Verification items for the finished model (mm, model axes). A direction names the side the tool comes from. Coordinates: 2 decimals unless noted, no trailing zeros. Loops run counter-clockwise (first coordinate to the right, second up) from the corner with the lowest first, then second, coordinate; pieces in that order, holes last.
Q1. Sectioned sample at D-D (y = 38). Enter the section's corners in (x, z).
Q2. Sectioned sample at B-B (x = 57). Enter the section's corners in (y, z).
Q3. Mould release check, pull along Y, two halves, no side actions. Record for faces 1 (the face through (58.49, 57.63, 1.48)), 2 (the face through (1, 2, 0)): +Y half, -Y half, draft (parallel to the pull), parting line (faces both ways), or undercut.
Q4. Sectioned sample at A-A (z = 0.5). Enter the section's corners in (x, y), then the cut area to 3 significant figures.
Q5. Sectioned sample at C-C (y = -12.5). Enter the section's corners in (x, z), then the cut area to 3 significant figures.
Q6. Go/stop test with a flat-tipped pin: P1, Ø1.5, axis at y = 7.5, z = 1, coming from the -X side. Record where the tip stops, or that it passes through.
Q7. Access from +Z, -Z, +X, -X, +Y, -Y to the whole of each face (thin tool, end or side, straight path). Record for faces 3 (the face through (-71.435, -78.018, 1.521)), 4 (the face through (1, 2, 3)), 5 (the face through (71.353, -77.767, 1.521)).
Q8. Material ranges on probe 1 along X at (y, z) = (-14, 0.35); probe 2 along Y at (x, z) = (48, 1.25); probe 3 along Y at (x, z) = (-61, 1.65), recorded low to high.
```python
from build123d import *

# Parameters (mm, degrees)
SALIENTE_EXTRUIR1_DEPTH = 3
REDONDEO1_R             = 30


with BuildPart() as part:
    # Croquis1 → Saliente-Extruir1 (new body)
    with BuildSketch(Plane.XY):
        Polygon((72.862780289, -137.153468779), (-72.862780289, -137.153468779), (-72.862780289, -77.415075694), (-43.862780289, -37.5), (-43.862780289, 37.5), (-72.862780289, 77.415075694), (-72.862780289, 137.153468779), (72.862780289, 137.153468779), (72.862780289, 77.415075694), (43.862780289, 37.5), (43.862780289, -37.5), (72.862780289, -77.415075694), align=None)
    extrude(amount=SALIENTE_EXTRUIR1_DEPTH)

    # Redondeo1
    redondeo1_edges = [part.edges().sort_by_distance(p)[0] for p in [
        (72.862780289, 77.415075694, 1.5),
        (43.862780289, 37.5, 1.5),
        (43.862780289, -37.5, 1.5),
        (72.862780289, -77.415075694, 1.5),
        (-72.862780289, -77.415075694, 1.5),
        (-43.862780289, -37.5, 1.5),
        (-43.862780289, 37.5, 1.5),
        (-72.862780289, 77.415075694, 1.5),
    ]]
    fillet(redondeo1_edges, radius=REDONDEO1_R)


solid = part.part
```
Geometry check:
1. outline: (-45.67, 0) - (45.67, 0) - (45.67, 3) - (-45.67, 3) - close
2. outline: (-137.15, 0) - (-55.58, 0) - (-55.58, 3) - (-137.15, 3) - close; (55.58, 0) - (137.15, 0) - (137.15, 3) - (55.58, 3) - close
3. face 1: undercut
3. face 2: draft
4. outline: (-72.86, -137.15) - (72.86, -137.15) - (72.86, -87.16) arc R30 ccw to (67.13, -69.53) - (49.59, -45.39) arc R30 cw to (43.86, -27.75) - (43.86, 27.75) arc R30 cw to (49.59, 45.39) - (67.13, 69.53) arc R30 ccw to (72.86, 87.16) - (72.86, 137.15) - (-72.86, 137.15) - (-72.86, 87.16) arc R30 ccw to (-67.13, 69.53) - (-49.59, 45.39) arc R30 cw to (-43.86, 27.75) - (-43.86, -27.75) arc R30 cw to (-49.59, -45.39) - (-67.13, -69.53) arc R30 ccw to (-72.86, -87.16) - close
4. area: 33,300 mm2
5. outline: (-43.86, 0) - (43.86, 0) - (43.86, 3) - (-43.86, 3) - close
5. area: 263 mm2
6. P1: stops at x = -43.86
7. face 3: +Z, -Z, -X
7. face 4: +Z, +X, -X, +Y, -Y
7. face 5: +Z, -Z, +X
8. probe 1: x = -43.86 to 43.86
8. probe 2: y = -137.15 to -42.95, 42.95 to 137.15
8. probe 3: y = -137.15 to -61.09, 61.09 to 137.15
